```python
from build123d import *

# Parameters (mm, degrees)
ESQUISSE1_W                                       = 12
ESQUISSE1_H                                       = 40
BOSS_EXTRU_1_DEPTH                                = 4
ESQUISSE2_W                                       = 12
ESQUISSE2_H                                       = 6
BOSS_EXTRU_2_DEPTH                                = 10
ESQUISSE3_R                                       = 1.6
ENL_V_MAT_EXTRU_1_DEPTH                           = 2
ESQUISSE4_W                                       = 12
ESQUISSE4_H                                       = 5
BOSS_EXTRU_3_DEPTH                                = 6
ESQUISSE5_R                                       = 0.95
ENL_V_MAT_EXTRU_2_DEPTH                           = 5
ESQUISSE6_W                                       = 10
ESQUISSE6_H                                       = 40
BOSS_EXTRU_4_DEPTH                                = 5
ESQUISSE7_R                                       = 2.5
ENL_V_MAT_EXTRU_3_DEPTH                           = 3
CHAMBRAGE_POUR_VIS_SIX_PANS_CREUX_M21_D           = 2.4
CHAMBRAGE_POUR_VIS_SIX_PANS_CREUX_M21_DEPTH       = 6
CHAMBRAGE_POUR_VIS_SIX_PANS_CREUX_M21_CBORE_D     = 4.4
CHAMBRAGE_POUR_VIS_SIX_PANS_CREUX_M21_CBORE_DEPTH = 2.4


with BuildPart() as part:
    # Esquisse1 → Boss.-Extru.1 (new body)
    with BuildSketch(Plane.XY):
        with Locations((4, 2.5)):
            Rectangle(ESQUISSE1_W, ESQUISSE1_H)
    extrude(amount=BOSS_EXTRU_1_DEPTH)

    # Esquisse2 → Boss.-Extru.2 (add)
    with BuildSketch(Plane(origin=(0, 0, 0), x_dir=(-1, 0, 0), z_dir=(0, 0, -1))):
        with Locations((-4, -14.5)):
            Rectangle(ESQUISSE2_W, ESQUISSE2_H)
    boss_extru_2 = extrude(amount=BOSS_EXTRU_2_DEPTH)

    # Symétrie1: Boss.-Extru.2 across plane
    add(boss_extru_2.mirror(Plane.ZX))

    # Esquisse3 → Enlèv. mat.-Extru.1 (cut)
    with BuildSketch(Plane.XY.offset(4)):
        with Locations((4, 10.6)):
            Circle(ESQUISSE3_R)
    extrude(amount=-ENL_V_MAT_EXTRU_1_DEPTH, mode=Mode.SUBTRACT)

    # Esquisse4 → Boss.-Extru.3 (add)
    with BuildSketch(Plane.XY.offset(4)):
        with Locations((4, 20)):
            Rectangle(ESQUISSE4_W, ESQUISSE4_H)
        with Locations((4, -15)):
            Rectangle(ESQUISSE4_W, ESQUISSE4_H)
    extrude(amount=BOSS_EXTRU_3_DEPTH)

    # Esquisse5 → Enlèv. mat.-Extru.2 (cut)
    with BuildSketch(Plane.XY.offset(10)):
        with Locations((4, -15)):
            Circle(ESQUISSE5_R)
        with Locations(Location((4, 20, 0), (0, 0, 180))):
            Circle(ESQUISSE5_R)
    extrude(amount=-ENL_V_MAT_EXTRU_2_DEPTH, mode=Mode.SUBTRACT)

    # Esquisse6 → Boss.-Extru.4 (add)
    with BuildSketch(Plane.ZY.offset(2)):
        with Locations((5, 2.5)):
            Rectangle(ESQUISSE6_W, ESQUISSE6_H)
    extrude(amount=BOSS_EXTRU_4_DEPTH)

    # Esquisse7 → Enlèv. mat.-Extru.3 (cut)
    with BuildSketch(Plane(origin=(-2, 0, 0), x_dir=(0, 0, -1), z_dir=(1, 0, 0))):
        with Locations(Location((-7, -5.7, 0), (0, 0, 90))):
            Circle(ESQUISSE7_R)
    extrude(amount=-ENL_V_MAT_EXTRU_3_DEPTH, mode=Mode.SUBTRACT)

    # Chambrage pour vis à six pans creux M21
    with Locations(Plane(origin=(0, -17.5, 0), x_dir=(-1, 0, 0), z_dir=(0, -1, 0))):
        with Locations((-5, 5)):
            chambrage_pour_vis_six_pans_creux_m21 = CounterBoreHole(CHAMBRAGE_POUR_VIS_SIX_PANS_CREUX_M21_D / 2, CHAMBRAGE_POUR_VIS_SIX_PANS_CREUX_M21_CBORE_D / 2, CHAMBRAGE_POUR_VIS_SIX_PANS_CREUX_M21_CBORE_DEPTH, depth=CHAMBRAGE_POUR_VIS_SIX_PANS_CREUX_M21_DEPTH)

    # Symétrie2: Chambrage pour vis à six pans creux M21 across plane
    add(chambrage_pour_vis_six_pans_creux_m21.mirror(Plane.ZX), mode=Mode.SUBTRACT)


solid = part.part
```
Build history of the part. All positions in model axes, mm. A direction names the side the tool comes from. Round coordinates to 2 decimals unless told otherwise and drop trailing zeros. Write each loop counter-clockwise with the first axis right and the second up, starting at its lowest first coordinate (ties: lowest second). Pieces come first, ordered by that corner, then holes. Notation, with made-up numbers: (5, -2) - (46, -2) arc R31 ccw to (46, 23) - close; hole circle Ø10 at (87, 48). An arc over 180 degrees is marked (long way). Answer as CSV lines item,"result".
Q1. Drill centre lines: probe 1 along Y at (x, z) = (4, 7.6); probe 2 along Y at (x, z) = (9.25, -7.5); probe 3 along X at (y, z) = (12.4, -5). Where is each one in solid material? Low to high. Write a range as [from, to].
Report:
probe 1,"y = [-17.5, -15.95], [-14.05, -12.5], [17.5, 19.05], [20.95, 22.5]"
probe 2,"y = [-17.5, -11.5], [11.5, 17.5]"
probe 3,"x = [-2, 3.8], [6.2, 10]"
Q2. Cut at C-C (z = -5). Write the cut outline in (x, y).
Report:
outline,"(-2, -17.5) - (2.8, -17.5) - (2.8, -15.1) - (3.8, -15.1) - (3.8, -11.5) - (-2, -11.5) - close; (-2, 11.5) - (3.8, 11.5) - (3.8, 15.1) - (2.8, 15.1) - (2.8, 17.5) - (-2, 17.5) - close; (6.2, -15.1) - (7.2, -15.1) - (7.2, -17.5) - (10, -17.5) - (10, -11.5) - (6.2, -11.5) - close; (6.2, 11.5) - (10, 11.5) - (10, 17.5) - (7.2, 17.5) - (7.2, 15.1) - (6.2, 15.1) - close"
Q3. Cut at A-A (z = -0.5). Write the cut outline in (x, y), and give its area (3 significant figures).
Report:
outline,"(-2, -17.5) - (10, -17.5) - (10, -11.5) - (-2, -11.5) - close; (-2, 11.5) - (10, 11.5) - (10, 17.5) - (-2, 17.5) - close"
area,"144 mm^2"
Q4. Drop flat-ended pins along their axis: pin 1 (5 mm diameter, centred on y = 14, z = -3.5, fed in from -X); pin 2 (2.5 mm diameter, centred on y = -4.5, z = 6.5, fed in from +X); pin 3 (3 mm diameter, centred on x = 7.5, z = -4, fed in from +Y); pin 4 (1.4 mm diameter, centred on x = 5, z = -5, fed in from +Y). Give the stop position or say it passes through.
Report:
pin 1,"stops at x = -2"
pin 2,"stops at x = -2"
pin 3,"stops at y = 17.5"
pin 4,"passes through"
Q5. Cut at D-D (x = 2). Write the cut outline in (y, z), and give its area (3 significant figures).
Report:
outline,"(-17.5, -10) - (-11.5, -10) - (-11.5, 0) - (11.5, 0) - (11.5, -10) - (17.5, -10) - (17.5, 0) - (22.5, 0) - (22.5, 10) - (17.5, 10) - (17.5, 4) - (-12.5, 4) - (-12.5, 10) - (-17.5, 10) - close"
area,"340 mm^2"
Q6. Pull direction X, two halves, no side cores. Call faces 1 (the cylindrical face through (2.9, -16.32, -5.66)), 2 (the cylindrical face through (-3.48, -4.55, 4.78)), 3 (the flat face through (-2, -15, -5)): +X half, -X half, draft (parallel to the pull), parting line (faces both ways), or undercut.
Report:
face 1,"undercut"
face 2,"draft"
face 3,"-X half"
Q7. Cut at B-B (y = -5.7). Write the cut outline in (x, z), and give its area (3 significant figures).
Report:
outline,"(-7, 0) - (10, 0) - (10, 4) - (-2, 4) - (-2, 4.5) - (-5, 4.5) - (-5, 9.5) - (-2, 9.5) - (-2, 10) - (-7, 10) - close"
area,"83.0 mm^2"
Q8. Tool access for faces 4 (the flat face through (-2, 3, 7)), 5 (the flat face through (-2, 14, -5)), 6 (the flat face through (4, -15.1, -4)), 7 (the cylindrical face through (5.526, 11.081, 3.014)): list every direction of +Z, -Z, +X, -X, +Y, -Y with a clear straight run to the whole face (end or side of a thin tool).
Report:
face 4,"+Z, +X"
face 5,"-Z, -X, +Y, -Y"
face 6,"-Y"
face 7,"+Z"
